```python
from build123d import *

# Parameters (mm, degrees)
SKETCH_1_R               = 1.275
EXTRUDE_1_DEPTH          = 6.4
FILLET_1_R               = 0.5
EXTRUDE_2_DEPTH          = 1.6
EXTRUDE_2_DEPTH_BACK     = 1.6
SKETCH_2_W               = 0.6
SKETCH_2_H               = 4.2
EXTRUDE_3_DEPTH          = 1.85
EXTRUDE_3_DEPTH_BACK     = 1.85
EXTRUDE_7_DEPTH          = 1.85
EXTRUDE_7_DEPTH_BACK     = 1.85
FILLET_2_R               = 0.5
FILLET_3_R               = 0.5
CUT_EXTRUDE_1_DEPTH      = 16.536582441
CUT_EXTRUDE_1_DEPTH_BACK = 16.536582441
SKETCH_5_R               = 0.8


with BuildPart() as part:
    # 草图1 → 凸台-拉伸1 (new body)
    with BuildSketch(Plane.XY):
        with BuildLine():
            Line((-10, -4.75), (-10, 4.75))
            Line((-10, 4.75), (-10, 4.95))
            ThreePointArc((-10, 4.95), (-9.853553391, 5.303553391), (-9.5, 5.45))
            Line((-9.5, 5.45), (-0.7, 5.45))
            Line((-0.7, 5.45), (0, 4.75))
            Line((0, 4.75), (10, 4.75))
            Line((10, 4.75), (10, -4.75))
            Line((10, -4.75), (6.025, -4.75))
            Line((6.025, -4.75), (5.825, -4.95))
            Line((5.825, -4.95), (3.675, -4.95))
            Line((3.675, -4.95), (3.475, -4.75))
            Line((3.475, -4.75), (-3.475, -4.75))
            Line((-3.475, -4.75), (-3.675, -4.95))
            Line((-3.675, -4.95), (-5.825, -4.95))
            Line((-5.825, -4.95), (-6.025, -4.75))
            Line((-6.025, -4.75), (-10, -4.75))
        make_face()
        with Locations((-4.75, -2.25)):
            Circle(SKETCH_1_R, mode=Mode.SUBTRACT)
        with Locations(Location((4.75, -2.25, 0), (0, 0, 180))):
            Circle(SKETCH_1_R, mode=Mode.SUBTRACT)
    extrude(amount=EXTRUDE_1_DEPTH)

    # 圆角1
    fillet_1_edges = [part.edges().sort_by_distance(p)[0] for p in [
        (10, 4.75, 3.2),
        (10, -4.75, 3.2),
        (-10, -4.75, 3.2),
    ]]
    fillet(fillet_1_edges, radius=FILLET_1_R)

    # 草图2 → 凸台-拉伸2 (add, two sides: drawn at the far end of the back side and taken through both)
    with BuildSketch(Plane.XY.offset(3.2).offset(-EXTRUDE_2_DEPTH_BACK)):
        with Locations((-8.05, -6.85)):
            Rectangle(SKETCH_2_W, SKETCH_2_H)
        with Locations((0.75, -6.85)):
            Rectangle(SKETCH_2_W, SKETCH_2_H)
        with Locations((8.05, -6.85)):
            Rectangle(SKETCH_2_W, SKETCH_2_H)
    extrude(amount=EXTRUDE_2_DEPTH + EXTRUDE_2_DEPTH_BACK)

    # 草图3 → 凸台-拉伸3 (add, two sides: drawn at the far end of the back side and taken through both)
    with BuildSketch(Plane.XY.offset(3.2).offset(-EXTRUDE_3_DEPTH_BACK)):
        with BuildLine():
            ThreePointArc((-3.75, 6.529795897), (-2.75, 6.95), (-1.75, 6.529795897))
            Line((-1.75, 6.529795897), (-1.75, 5.45))
            Line((-1.75, 5.45), (-3.75, 5.45))
            Line((-3.75, 5.45), (-3.75, 6.529795897))
        make_face()
    extrude(amount=EXTRUDE_3_DEPTH + EXTRUDE_3_DEPTH_BACK)

    # 草图4 → 凸台-拉伸7 (add, two sides: drawn at the far end of the back side and taken through both)
    with BuildSketch(Plane.XY.offset(3.2).offset(-EXTRUDE_7_DEPTH_BACK)):
        Polygon((-2.796894142, 8.076477611), (-6.875, 7.398937263), (-6.875, 5.45), (-6.875, 4.395314544), (-5.875, 4.395314544), (-5.875, 5.45), (-5.875, 6.45), (-5.875, 6.551370746), (9.072540681, 9.03476923), (8.908646315, 10.021247125), align=None)
    extrude(amount=EXTRUDE_7_DEPTH + EXTRUDE_7_DEPTH_BACK)

    # 圆角2
    fillet_2_edges = [part.edges().sort_by_distance(p)[0] for p in [
        (-5.875, 6.551370746, 3.2),
        (8.990593498, 9.528008177, 5.05),
        (-6.875, 7.398937263, 3.2),
        (8.990593498, 9.528008177, 1.35),
    ]]
    fillet(fillet_2_edges, radius=FILLET_2_R)

    # 圆角3
    fillet_3_edges = [part.edges().sort_by_distance(p)[0] for p in [
        (-8.05, -8.95, 1.6),
        (-8.05, -8.95, 4.8),
        (0.75, -8.95, 1.6),
        (0.75, -8.95, 4.8),
        (8.05, -8.95, 1.6),
        (8.05, -8.95, 4.8),
    ]]
    fillet(fillet_3_edges, radius=FILLET_3_R)

    # 草图5 → 切除-拉伸1 (cut, two sides: drawn at the far end of the back side and taken through both)
    with BuildSketch(Plane(origin=(0, 0, 0), x_dir=(0, 0, -1), z_dir=(1, 0, 0)).offset(-CUT_EXTRUDE_1_DEPTH_BACK)):
        with Locations((-3.2, -7.35)):
            Circle(SKETCH_5_R)
    extrude(amount=CUT_EXTRUDE_1_DEPTH + CUT_EXTRUDE_1_DEPTH_BACK, mode=Mode.SUBTRACT)


solid = part.part
```
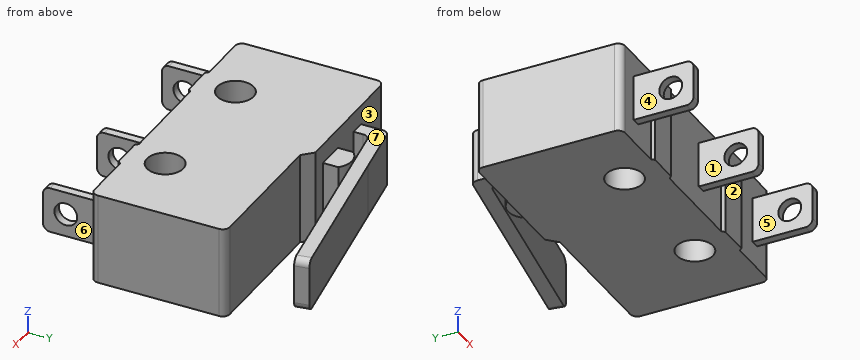
Could you check a few things on this model? Use its own coordinates, in mm. Face numbers are marked on the shaded views. A direction names the side the tool comes from. Coordinates: 2 decimals unless noted, no trailing zeros. Loops run counter-clockwise (first coordinate to the right, second up) from the corner with the lowest first, then second, coordinate; pieces in that order, holes last. Notation, with made-up numbers: M -11,51 L 0,51 A16 cw 0,61 Z; hole C 89.25,-8.5 d8. An arc over 180 degrees is marked long. Put each result on its own line as item: value. Start each with the question number.
(1) Suppose I cut it at D-D on y = -2.25. Please give me the cut outline in (x, z) (3 decimals), then the cut area to 3 significant figures.
(2) For the marked faces 4, 5, 6 and 7, which set-ups out of +Z, -Z, +X, -X, +Y, -Y let a thin tool reach every point of the face, with its end or its side?
(3) Thinking about a two-plate mould opening in Y: for the marked faces 1, 2 and 3, which applies, pulls with the +Y half, pulls with the -Y half, needs draft (parallel to the pull), parting line crosses it, or undercut?
(4) Suppose I cut it at B-B on z = 5.5. Please give me the cut outline in (x, y) (3 decimals), then the cut area to 3 significant figures.
(5) Suppose I cut it at C-C on x = 4.75. Please give me the cut outline in (y, z) (3 decimals).
(6) I need wall thicknesses on line 1 (Z direction, x = -8, y = -7.35); line 2 (X direction, y = -7.5, z = 4.5); line 3 (Y direction, x = -5.25, z = 4.5). Which ranges of each line are inside material? Lowest first, please. Write a range as from..to.
(7) Will these pins go through, and if not, where does the flat tip stop? P1, Ø1.2, axis at x = -2.5, y = 6, coming from the +Z side; P2, Ø0.6, axis at x = 5, z = 2, coming from the -Y side; P3, Ø3.5, axis at y = -7.5, z = 3.5, coming from the +X side; P4, Ø1, axis at y = -6, z = 2.5, coming from the -X side.
(8) Suppose I cut it at A-A on y = 5.75. Please give me the cut outline in (x, z) (3 decimals).
Solutions:
1. outline: M -10,0 L -6.025,0 L -6.025,6.4 L -10,6.4 Z; M -3.475,0 L 3.475,0 L 3.475,6.4 L -3.475,6.4 Z; M 6.025,0 L 10,0 L 10,6.4 L 6.025,6.4 Z
1. area: 95.4 mm2
2. face 4: +Z, -Z, -X, -Y
2. face 5: +Z, -Z, -Y
2. face 6: +Z, -Z, +X, -Y
2. face 7: +Z, +X, -X, +Y
3. face 1: needs draft
3. face 2: pulls with the -Y half
3. face 3: undercut
4. outline: M -10,-4.25 A0.5 ccw -9.5,-4.75 L -6.025,-4.75 L -5.825,-4.95 L -3.675,-4.95 L -3.475,-4.75 L 3.475,-4.75 L 3.675,-4.95 L 5.825,-4.95 L 6.025,-4.75 L 9.5,-4.75 A0.5 ccw 10,-4.25 L 10,4.25 A0.5 ccw 9.5,4.75 L 0,4.75 L -0.7,5.45 L -9.5,5.45 A0.5 ccw -10,4.95 Z; hole C -4.75,-2.25 d2.55; hole C 4.75,-2.25 d2.55
4. area: 187 mm2
5. outline: M -4.95,0 L -3.525,0 L -3.525,6.4 L -4.95,6.4 Z; M -0.975,0 L 4.75,0 L 4.75,6.4 L -0.975,6.4 Z; M 8.317,1.35 L 9.33,1.35 L 9.33,5.05 L 8.317,5.05 Z
6. line 1: z = 1.6..2.4, 4..4.8
6. line 2: x = -8.35..-7.75, 0.45..1.05, 7.75..8.35
6. line 3: y = -4.95..-3.42, -1.08..5.45, 6.66..7.67
7. P1: stops at z = 6.4
7. P2: stops at y = -4.95
7. P3: stops at x = 8.35
7. P4: stops at x = -8.35
8. outline: M -6.875,1.35 L -5.875,1.35 L -5.875,5.05 L -6.875,5.05 Z; M -3.75,1.35 L -1.75,1.35 L -1.75,5.05 L -3.75,5.05 Z
